from build123d import *

# Parameters (mm, degrees)
BOSS_EXTRUDE1_DEPTH = 45.72
SKETCH2_R           = 12.446
CUT_EXTRUDE1_DEPTH  = 112.086312694
SKETCH3_R           = 1.5748
CUT_EXTRUDE2_DEPTH  = 112.086312694
SKETCH4_R           = 1.9558
CUT_EXTRUDE3_DEPTH  = 45.72


with BuildPart() as part:
    # Sketch1 → Boss-Extrude1 (new body)
    with BuildSketch(Plane.XY):
        with BuildLine():
            Line((0, 0), (18.796, 0))
            ThreePointArc((18.796, 0), (20.592051224, 0.743948776), (21.336, 2.54))
            Line((21.336, 2.54), (21.336, 43.942))
            ThreePointArc((21.336, 43.942), (22.079948776, 45.738051224), (23.876, 46.482))
            Line((23.876, 46.482), (65.532, 46.482))
            ThreePointArc((65.532, 46.482), (67.328051224, 45.738051224), (68.072, 43.942))
            Line((68.072, 43.942), (68.072, 2.54))
            ThreePointArc((68.072, 2.54), (68.815948776, 0.743948776), (70.612, 0))
            Line((70.612, 0), (89.408, 0))
            Line((89.408, 0), (89.408, 1.016))
            Line((89.408, 1.016), (70.612, 1.016))
            ThreePointArc((70.612, 1.016), (69.534369265, 1.462369265), (69.088, 2.54))
            Line((69.088, 2.54), (69.088, 43.942))
            ThreePointArc((69.088, 43.942), (68.046471714, 46.456471714), (65.532, 47.498))
            Line((65.532, 47.498), (23.876, 47.498))
            ThreePointArc((23.876, 47.498), (21.361528286, 46.456471714), (20.32, 43.942))
            Line((20.32, 43.942), (20.32, 2.54))
            ThreePointArc((20.32, 2.54), (19.873630735, 1.462369265), (18.796, 1.016))
            Line((18.796, 1.016), (0, 1.016))
            Line((0, 1.016), (0, 0))
        make_face()
    extrude(amount=BOSS_EXTRUDE1_DEPTH)

    # Sketch2 → Cut-Extrude1 (cut, through all)
    with BuildSketch(Plane(origin=(0, 47.498, 0), x_dir=(1, 0, 0), z_dir=(0, 1, 0))):
        with Locations(Location((44.704, -22.86, 0), (0, 0, 270))):
            Circle(SKETCH2_R)
    extrude(amount=-CUT_EXTRUDE1_DEPTH, mode=Mode.SUBTRACT)

    # Sketch3 → Cut-Extrude2 (cut, through all)
    with BuildSketch(Plane(origin=(0, 47.498, 0), x_dir=(1, 0, 0), z_dir=(0, 1, 0))):
        with Locations(Location((58.936729391, -7.238711644, 0), (0, 0, 270))):
            Circle(SKETCH3_R)
        with Locations(Location((30.471270609, -7.238711644, 0), (0, 0, 270))):
            Circle(SKETCH3_R)
        with Locations(Location((58.936729391, -38.481288356, 0), (0, 0, 270))):
            Circle(SKETCH3_R)
        with Locations(Location((30.471270609, -38.481288356, 0), (0, 0, 270))):
            Circle(SKETCH3_R)
    extrude(amount=-CUT_EXTRUDE2_DEPTH, mode=Mode.SUBTRACT)

    # Sketch4 → Cut-Extrude3 (cut)
    with BuildSketch(Plane(origin=(0, 1.016, 0), x_dir=(1, 0, 0), z_dir=(0, 1, 0))):
        with Locations(Location((10.7188, -7.5438, 0), (0, 0, 270))):
            Circle(SKETCH4_R)
        with Locations(Location((10.7188, -23.749, 0), (0, 0, 270))):
            Circle(SKETCH4_R)
        with Locations(Location((10.7188, -39.9542, 0), (0, 0, 270))):
            Circle(SKETCH4_R)
    cut_extrude3 = extrude(amount=-CUT_EXTRUDE3_DEPTH, mode=Mode.SUBTRACT)

    # Mirror1: Cut-Extrude3 across plane
    add(cut_extrude3.mirror(Plane.ZY.offset(-44.704)), mode=Mode.SUBTRACT)


solid = part.part
Model file for the job. Use its own axes, mm. A direction names the side the tool comes from. Give positions to 0.01 mm unless a question says otherwise; leave off trailing zeros. Order: outer loops, then holes, each group sorted by start corner. A loop starts at its lowest first (then second) coordinate and runs counter-clockwise, first axis right, second up. Notation, with made-up numbers: M 84.25,12.5 L 135.25,12.5 A23 cw 135.25,21.5 Z; hole C 75,47.25 d4. An arc over 180 degrees is marked long. Put each result on its own line as item: value. Start each with the question number.
(1) Band-saw the part on A-A on y = 33.5. Give the cut face in (x, z), then the cut area to 3 significant figures.
(2) Band-saw the part on C-C on z = 22.86. Count the separate pieces of the cut face and the enclosed holes in it, then the cut area to 3 significant figures.
(3) Band-saw the part on B-B on x = 49. Give the cut face in (y, z).
(4) Drill centre lines: L1, parallel to X at y = 21, z = 8; L2, parallel to Y at x = 6.5, z = 23; L3, parallel to Y at x = 65, z = 18. Where is each one in solid material? Low to high. Write a range as [from, to].
(5) Band-saw the part on D-D on x = 75. Give the cut face in (y, z).
(6) Pin check, flat tips, straight feed: pin 1 Ø5 at (x, z) = (10.72, 23.75) entering from +Y; pin 2 Ø1.5 at (y, z) = (32.5, 7) entering from -X; pin 3 Ø4 at (x, z) = (27.5, 31.5) entering from -Y; pin 4 Ø2.5 at (x, z) = (30.47, 38.48) entering from +Y. Stop position of each tip, or through.
(7) Pull direction Z, two halves, no side cores. Call faces 1 (the face through (68.1, 46.4, 22.5)), 2 (the face through (57.4, 47, 6.9)), 3 (the face through (21, 26, 45.72)): released by +Z, released by -Z, zero draft, split by the parting line, or undercut.
(8) Tool access for faces 4 (the face through (8.81, 0.52, 7.12)), 5 (the face through (20.57, 0.72, 22.54)), 6 (the face through (82, 1.016, 23)), 7 (the face through (7, 1.016, 23)): list every direction of +Z, -Z, +X, -X, +Y, -Y with a clear straight run to the whole face (end or side of a thin tool).
Results below:
1. outline: M 20.32,0 L 21.34,0 L 21.34,45.72 L 20.32,45.72 Z; M 68.07,0 L 69.09,0 L 69.09,45.72 L 68.07,45.72 Z
1. area: 92.9 mm2
2. separate pieces: 4
2. enclosed holes: 0
2. area: 148 mm2
3. outline: M 46.48,0 L 47.5,0 L 47.5,11.18 L 46.48,11.18 Z; M 46.48,34.54 L 47.5,34.54 L 47.5,45.72 L 46.48,45.72 Z
4. L1: x = [20.32, 21.34], [68.07, 69.09]
4. L2: y = [0, 1.02]
4. L3: y = [46.48, 47.5]
5. outline: M 0,0 L 1.02,0 L 1.02,45.72 L 0,45.72 Z
6. pin 1: stops at y = 1.02
6. pin 2: stops at x = 20.32
6. pin 3: stops at y = 46.48
6. pin 4: passes through
7. face 1: zero draft
7. face 2: undercut
7. face 3: released by +Z
8. face 4: +Y, -Y
8. face 5: +Z, -Z, -Y
8. face 6: +Z, -Z, +X, +Y
8. face 7: +Z, -Z, -X, +Y
